CAD build for the part. Positions are in the model's coordinates, mm. A direction names the side the tool comes from. Round coordinates to 2 decimals unless told otherwise and drop trailing zeros. Loops run counter-clockwise (first coordinate to the right, second up) from the corner with the lowest first, then second, coordinate; pieces in that order, holes last.
```python
from build123d import *

# Parameters (mm, degrees)
SKICA1_R                 = 4
SKICA1_W                 = 1.7
SKICA1_H                 = 7.8
SKICA1_R_2               = 1.5
P_IDAT_VYSUNUT_M3_DEPTH  = 1.4
SKICA3_R                 = 3.986213299
ODEBRAT_VYSUNUT_M1_DEPTH = 0.9


with BuildPart() as part:
    # Skica1 → P_idat vysunut_m3 (new body)
    # profile 1 of 3: a face of its own
    with BuildSketch(Plane.XY):
        with BuildLine():
            ThreePointArc((-11.45, -6.25), (-11.803553391, -6.103553391), (-11.95, -5.75))
            Line((-11.95, -5.75), (-11.95, 3.25))
            ThreePointArc((-11.95, 3.25), (-11.071320344, 5.371320344), (-8.95, 6.25))
            Line((-8.95, 6.25), (8.95, 6.25))
            ThreePointArc((8.95, 6.25), (11.071320344, 5.371320344), (11.95, 3.25))
            Line((11.95, 3.25), (11.95, -5.75))
            ThreePointArc((11.95, -5.75), (11.803553391, -6.103553391), (11.45, -6.25))
            Line((11.45, -6.25), (-11.45, -6.25))
        make_face()
        with Locations((-6, 0.95)):
            Circle(SKICA1_R, mode=Mode.SUBTRACT)
        with Locations((6, 0.95)):
            Circle(SKICA1_R, mode=Mode.SUBTRACT)
        Rectangle(SKICA1_W, SKICA1_H, mode=Mode.SUBTRACT)
    # profile 2 of 3: a face of its own
    with BuildSketch(Plane.XY):
        with Locations((-6, 0.95)):
            Circle(SKICA1_R)
        with Locations((-6, 0.95)):
            Circle(SKICA1_R_2, mode=Mode.SUBTRACT)
    # profile 3 of 3: a face of its own
    with BuildSketch(Plane.XY):
        with Locations((6, 0.95)):
            Circle(SKICA1_R)
        with Locations((6, 0.95)):
            Circle(SKICA1_R_2, mode=Mode.SUBTRACT)
    extrude(amount=P_IDAT_VYSUNUT_M3_DEPTH)

    # Skica3 → Odebrat vysunut_m1 (cut)
    with BuildSketch(Plane(origin=(0, 0, 0), x_dir=(-1, 0, 0), z_dir=(0, 0, -1))):
        with Locations((-6, 0.95)):
            Circle(SKICA3_R)
        with Locations((6, 0.95)):
            Circle(SKICA3_R)
    extrude(amount=-ODEBRAT_VYSUNUT_M1_DEPTH, mode=Mode.SUBTRACT)


solid = part.part
```
Item 1: Two-plate mould, pull along X, no slides. Class faces 4 (the flat face through (0, -6.25, 1)), 5 (the flat face through (0.85, 0, 1)), 6 (the cylindrical face through (-7.5, 1, 1.1)), 7 (the flat face through (-11.95, -1, 1)): released by +X, released by -X, zero draft, split by the parting line, or undercut.
Answers follow:
face 4: zero draft
face 5: undercut
face 6: undercut
face 7: released by -X
Item 2: Cut at B-B, the plane y = 0.95. Give the cut face in (x, z), plus the area to 3 significant figures.
Answers follow:
outline: (-11.95, 0) - (-9.99, 0) - (-9.99, 0.9) - (-7.5, 0.9) - (-7.5, 1.4) - (-11.95, 1.4) - close; (-4.5, 0.9) - (-2.01, 0.9) - (-2.01, 0) - (-0.85, 0) - (-0.85, 1.4) - (-4.5, 1.4) - close; (0.85, 0) - (2.01, 0) - (2.01, 0.9) - (4.5, 0.9) - (4.5, 1.4) - (0.85, 1.4) - close; (7.5, 0.9) - (9.99, 0.9) - (9.99, 0) - (11.95, 0) - (11.95, 1.4) - (7.5, 1.4) - close
area: 13.7 mm2
Item 3: Flat gauge pin, fed straight in: P1, Ø2.5, axis at x = 6, y = 1.5, coming from the -Z side. Where does the tip first touch, or does it go through?
Answers follow:
P1: stops at z = 0.9
Item 4: Cut at D-D, the plane x = 3.5. Give the cut face in (y, z), plus the area to 3 significant figures.
Answers follow:
outline: (-6.25, 0) - (-2.15, 0) - (-2.15, 0.9) - (4.05, 0.9) - (4.05, 0) - (6.25, 0) - (6.25, 1.4) - (-6.25, 1.4) - close
area: 11.9 mm2
Item 5: Probe line 1 (X direction, y = 0.95, z = 1.35); line 2 (Y direction, x = 6, z = 1.1); line 3 (Y direction, x = -0.5, z = 1.35). List the from-to ranges inside material, lowest first.
Answers follow:
line 1: x = -11.95 to -7.5, -4.5 to -0.85, 0.85 to 4.5, 7.5 to 11.95
line 2: y = -6.25 to -0.55, 2.45 to 6.25
line 3: y = -6.25 to -3.9, 3.9 to 6.25
Item 6: Cut at A-A, the plane x = -6. Give the cut face in (y, z).
Answers follow:
outline: (-6.25, 0) - (-3.04, 0) - (-3.04, 0.9) - (-0.55, 0.9) - (-0.55, 1.4) - (-6.25, 1.4) - close; (2.45, 0.9) - (4.94, 0.9) - (4.94, 0) - (6.25, 0) - (6.25, 1.4) - (2.45, 1.4) - close
Item 7: Cut at C-C, the plane x = -0.25. Give the cut face in (y, z).
Answers follow:
outline: (-6.25, 0) - (-3.9, 0) - (-3.9, 1.4) - (-6.25, 1.4) - close; (3.9, 0) - (6.25, 0) - (6.25, 1.4) - (3.9, 1.4) - close
Item 8: 3-axis set-ups, long thin cutter, end or side, ignore diameter. For faces 1 (the flat face through (-0.85, 0, 1)), 2 (the flat face through (6, -1, 0.9)), 3 (the flat face through (2, -1, 0)): which of +Z, -Z, +X, -X, +Y, -Y reach the whole face in a straight line?
Answers follow:
face 1: +Z, -Z
face 2: -Z
face 3: -Z, +X, -X, +Y, -Y
